from build123d import *

# Parameters (mm, degrees)
SKETCH1_W                = 340
SKETCH1_H                = 210
BOSS_EXTRUDE1_DEPTH      = 320
SKETCH2_W                = 300
SKETCH2_H                = 170
CUT_EXTRUDE1_DEPTH       = 378.259857393
SKETCH3_W                = 300
SKETCH3_H                = 600
CUT_EXTRUDE2_DEPTH       = 419.807831827
SKETCH4_W                = 170
SKETCH4_H                = 600
CUT_EXTRUDE3_DEPTH       = 479.565564996
BOSS_EXTRUDE2_DEPTH      = 152.5
BOSS_EXTRUDE2_DEPTH_BACK = 152.5
SKETCH5_W                = 20
SKETCH5_H                = 20
SKETCH5_W_2              = 40
SKETCH6_W                = 20
SKETCH6_H                = 305
CUT_EXTRUDE4_DEPTH       = 403.189321091


with BuildPart() as part:
    # Sketch1 → Boss-Extrude1 (new body)
    with BuildSketch(Plane(origin=(0, 0, 0), x_dir=(1, 0, 0), z_dir=(0, 1, 0))):
        Rectangle(SKETCH1_W, SKETCH1_H)
    extrude(amount=-BOSS_EXTRUDE1_DEPTH)

    # Sketch2 → Cut-Extrude1 (cut, through all)
    with BuildSketch(Plane(origin=(0, 0, 0), x_dir=(1, 0, 0), z_dir=(0, 1, 0))):
        Rectangle(SKETCH2_W, SKETCH2_H)
    extrude(amount=-CUT_EXTRUDE1_DEPTH, mode=Mode.SUBTRACT)

    # Sketch3 → Cut-Extrude2 (cut, through all)
    with BuildSketch(Plane.XY.offset(105)):
        with Locations((0, -320)):
            Rectangle(SKETCH3_W, SKETCH3_H)
    extrude(amount=-CUT_EXTRUDE2_DEPTH, mode=Mode.SUBTRACT)

    # Sketch4 → Cut-Extrude3 (cut, through all)
    with BuildSketch(Plane(origin=(170, 0, 0), x_dir=(0, 0, -1), z_dir=(1, 0, 0))):
        with Locations((0, -320)):
            Rectangle(SKETCH4_W, SKETCH4_H)
    extrude(amount=-CUT_EXTRUDE3_DEPTH, mode=Mode.SUBTRACT)

    # Sketch5 → Boss-Extrude2 (add, two sides: drawn at the far end of the back side and taken through both)
    with BuildSketch(Plane.XY.offset(-BOSS_EXTRUDE2_DEPTH_BACK)):
        with Locations((-160, -330)):
            Rectangle(SKETCH5_W, SKETCH5_H)
        with Locations((170, -330)):
            Rectangle(SKETCH5_W_2, SKETCH5_H)
    extrude(amount=BOSS_EXTRUDE2_DEPTH + BOSS_EXTRUDE2_DEPTH_BACK)

    # Sketch6 → Cut-Extrude4 (cut, through all)
    with BuildSketch(Plane(origin=(0, -320, 0), x_dir=(1, 0, 0), z_dir=(0, 1, 0))):
        with Locations((180, 0)):
            Rectangle(SKETCH6_W, SKETCH6_H)
    extrude(amount=-CUT_EXTRUDE4_DEPTH, mode=Mode.SUBTRACT)


solid = part.part
Read the model definition and answer for the solid it produces. Units are mm, in the model's axes. A direction names the side the tool comes from. Give positions to 0.01 mm unless a question says otherwise; leave off trailing zeros. Write each loop counter-clockwise with the first axis right and the second up, starting at its lowest first coordinate (ties: lowest second). Pieces come first, ordered by that corner, then holes. Notation, with made-up numbers: (69.25, -11) - (73.25, -11) arc R20 ccw to (73.25, 10) - close; hole circle Ø3 at (-26.5, -6). An arc over 180 degrees is marked (long way). Return JSON: item names as keys, results as strings.
Q1. A cutting plane is placed at D-D, the plane z = 120. Determine the outline of the cut face in (x, y), and give its area (3 significant figures).
Reply:
{"outline": "(-170, -340) - (-150, -340) - (-150, -320) - (-170, -320) - close; (150, -340) - (170, -340) - (170, -320) - (150, -320) - close", "area": "800 mm²"}
Q2. A cutting plane is placed at A-A, the plane x = -102.5. Determine the outline of the cut face in (y, z), and give its area (3 significant figures).
Reply:
{"outline": "(-20, -105) - (0, -105) - (0, -85) - (-20, -85) - close; (-20, 85) - (0, 85) - (0, 105) - (-20, 105) - close", "area": "800 mm²"}
Q3. Given P1, Ø10, axis at x = -82.5, z = -97.5, coming from the +Y side; P2, Ø6, axis at x = -161.5, z = 136, coming from the +Y side; P3, Ø16, axis at x = 64, y = -13, coming from the -Z side; P4, Ø10, axis at x = 44, z = 91, coming from the -Y side, each flat-ended and moving along its own axis, determine where each tip first touches the part or whether it passes through.
Reply:
{"P1": "y = 0", "P2": "y = -320", "P3": "z = -105", "P4": "y = -20"}
Q4. A cutting plane is placed at C-C, the plane y = -65. Determine the outline of the cut face in (x, z), and give its area (3 significant figures).
Reply:
{"outline": "(-170, -105) - (-150, -105) - (-150, -85) - (-170, -85) - close; (-170, 85) - (-150, 85) - (-150, 105) - (-170, 105) - close; (150, -105) - (170, -105) - (170, -85) - (150, -85) - close; (150, 85) - (170, 85) - (170, 105) - (150, 105) - close", "area": "1,600 mm²"}
Q5. A cutting plane is placed at B-B, the plane z = -53. Determine the outline of the cut face in (x, y), and give its area (3 significant figures).
Reply:
{"outline": "(-170, -340) - (-150, -340) - (-150, -320) - (-170, -320) - close; (-170, -20) - (-150, -20) - (-150, 0) - (-170, 0) - close; (150, -340) - (170, -340) - (170, -320) - (150, -320) - close; (150, -20) - (170, -20) - (170, 0) - (150, 0) - close", "area": "1,600 mm²"}
Q6. For faces 4 (the face through (160, -320, -129)), 5 (the face through (-150, -10, 1)), 6 (the face through (160, -172, -85)), 7 (the face through (150, -216, -90)), determine the directions among +Z, -Z, +X, -X, +Y, -Y from which every point of the face is accessible in a straight line to the end or side of a thin tool.
Reply:
{"face 4": "-Z, +X, -X, +Y", "face 5": "+Y, -Y", "face 6": "+X, -X", "face 7": "+Z, -Z, -Y"}
Q7. For a pull along Z with two mould halves and no side action, classify faces 1 (the face through (-160, -172, -85)), 2 (the face through (160, -330, -152.5)), 3 (the face through (-170, -183, -91)) as released by +Z, released by -Z, zero draft, split by the parting line, or undercut.
Reply:
{"face 1": "undercut", "face 2": "released by -Z", "face 3": "zero draft"}
Q8. Consider line 1 along X through (y, z) = (-100, -94); line 2 along Y through (x, z) = (-155.5, -83.5); line 3 along Y through (x, z) = (24, 94). Determine where each line is inside the solid, lowest interval first. Write a range as [from, to].
Reply:
{"line 1": "[-170, -150], [150, 170]", "line 2": "[-340, -320], [-20, 0]", "line 3": "[-20, 0]"}
